Model file for the job. Use its own axes, mm. Face numbers are marked on the shaded views. A direction names the side the tool comes from. Coordinates: 2 decimals unless noted, no trailing zeros. Write each loop counter-clockwise with the first axis right and the second up, starting at its lowest first coordinate (ties: lowest second). Pieces come first, ordered by that corner, then holes. Notation, with made-up numbers: (-17, -3) - (23, -3) arc R27 ccw to (23, 26) - close; hole circle Ø9 at (14.25, -9.5). An arc over 180 degrees is marked (long way). Put each result on its own line as item: value. Start each with the question number.
1. Drop flat-ended pins along their axis: P1, Ø2.5, axis at y = 7.5, z = 43.5, coming from the +X side; P2, Ø1.6, axis at y = 60.5, z = 43.5, coming from the -X side. Give the stop position or say it passes through.
2. Saw through at B-B, the plane z = 30. Write the cut outline in (x, y).
3. Saw through at D-D, the plane z = 13.5. Write the cut outline in (x, y).
4. Saw through at A-A, the plane x = 66. Write the cut outline in (y, z).
5. Drill centre lines: L1, parallel to Y at x = 2.55, z = 43.5; L2, parallel to X at y = 42, z = 26.5; L3, parallel to Z at x = 103.3, y = 7.5. Where is each one in solid material? Low to high. Write a range as from..to.
6. Pull direction X, two halves, no side cores. Call the marked faces 1, 2 and 3: released by +X, released by -X, zero draft, split by the parting line, or undercut.
7. Which spindle directions (+Z, -Z, +X, -X, +Y, -Y) get a long thin tool onto all of the face, cutting with end or side? Do the marked faces 4 and 5. Say none if no direction does.
8. Saw through at C-C, the plane z = 4.5. Write the cut outline in (x, y), plus the area to 3 significant figures.
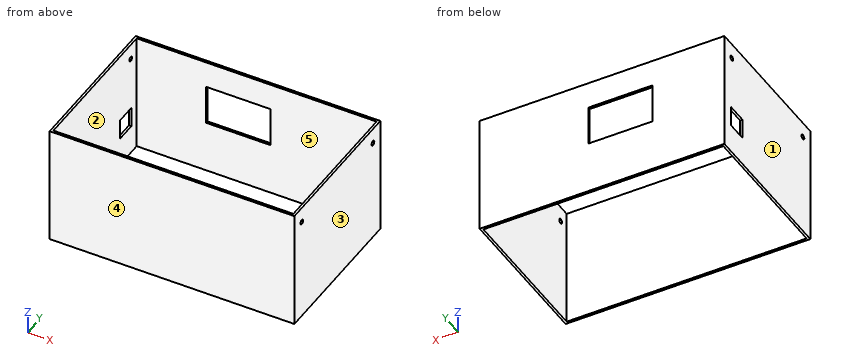
```python
from build123d import *

# Parameters (mm, degrees)
SKETCH_1_W               = 102
SKETCH_1_H               = 64
SKETCH_1_W_2             = 100
SKETCH_1_H_2             = 62
EXTRUDE_1_DEPTH          = 50
CUT_EXTRUDE_2_DEPTH      = 102
CUT_EXTRUDE_2_DEPTH_BACK = 1
SKETCH_5_R               = 1
SKETCH_7_W               = 8.5
SKETCH_7_H               = 8.5
CUT_EXTRUDE_4_DEPTH      = 10
SKETCH_8_W               = 26.7
SKETCH_8_H               = 16.7
CUT_EXTRUDE_5_DEPTH      = 10


with BuildPart() as part:
    # Эскиз1 → Бобышка-Вытянуть1 (new body)
    with BuildSketch(Plane.XY):
        with Locations((53, 34)):
            Rectangle(SKETCH_1_W, SKETCH_1_H)
        with Locations((53, 34)):
            Rectangle(SKETCH_1_W_2, SKETCH_1_H_2, mode=Mode.SUBTRACT)
    extrude(amount=EXTRUDE_1_DEPTH)

    # Эскиз5 → Вырез-Вытянуть2 (cut, two sides: drawn at the far end of the back side and taken through both)
    with BuildSketch(Plane.ZY.offset(-103).offset(-CUT_EXTRUDE_2_DEPTH_BACK)):
        with Locations((43.5, 7.5)):
            Circle(SKETCH_5_R)
        with Locations((43.5, 60.5)):
            Circle(SKETCH_5_R)
    extrude(amount=CUT_EXTRUDE_2_DEPTH + CUT_EXTRUDE_2_DEPTH_BACK, mode=Mode.SUBTRACT)

    # Эскиз7 → Вырез-Вытянуть4 (cut)
    with BuildSketch(Plane.ZY.offset(-2)):
        with Locations((16.25, 56.75)):
            Rectangle(SKETCH_7_W, SKETCH_7_H)
    extrude(amount=-CUT_EXTRUDE_4_DEPTH, mode=Mode.SUBTRACT)

    # Эскиз8 → Вырез-Вытянуть5 (cut)
    with BuildSketch(Plane(origin=(0, 66, 0), x_dir=(1, 0, 0), z_dir=(0, 1, 0))):
        with Locations((45.35, -30.35)):
            Rectangle(SKETCH_8_W, SKETCH_8_H)
    extrude(amount=-CUT_EXTRUDE_5_DEPTH, mode=Mode.SUBTRACT)


solid = part.part
```
Final values:
1. P1: stops at x = 104
1. P2: passes through
2. outline: (2, 2) - (104, 2) - (104, 66) - (58.7, 66) - (58.7, 65) - (103, 65) - (103, 3) - (3, 3) - (3, 65) - (32, 65) - (32, 66) - (2, 66) - close
3. outline: (2, 2) - (104, 2) - (104, 66) - (2, 66) - (2, 61) - (3, 61) - (3, 65) - (103, 65) - (103, 3) - (3, 3) - (3, 52.5) - (2, 52.5) - close
4. outline: (2, 0) - (3, 0) - (3, 50) - (2, 50) - close; (65, 0) - (66, 0) - (66, 50) - (65, 50) - close
5. L1: y = 2..6.5, 8.5..59.5, 61.5..66
5. L2: x = 2..3, 103..104
5. L3: z = 0..42.5, 44.5..50
6. face 1: released by -X
6. face 2: undercut
6. face 3: released by +X
7. face 4: +Z, -Z, +X, -X, -Y
7. face 5: +Z, -Z
8. outline: (2, 2) - (104, 2) - (104, 66) - (2, 66) - close; hole (3, 3) - (103, 3) - (103, 65) - (3, 65) - close
8. area: 328 mm²
